Verification items for the finished model (mm, model axes). Round coordinates to 2 decimals unless told otherwise and drop trailing zeros. Write each loop counter-clockwise with the first axis right and the second up, starting at its lowest first coordinate (ties: lowest second). Pieces come first, ordered by that corner, then holes. Notation, with made-up numbers: (13.25, 85.25) -> (25.25, 85.25) arc R29 ccw to (25.25, 116.25) -> close; hole circle Ø1 at (38.25, 26.5). An arc over 180 degrees is marked (long way). Use CSV: the item, a comma, the result in double quotes.
Solid Edge part; units mm, degrees
sketch "Sketch1" plane through (0, 0, 0) normal (0, 0, 1) x (1, 0, 0)
  circle A0 centre (0, 0) radius 4.5
  circle A1 centre (0, 0) radius 2.6
extrude "Protrusion1" add sketch "Sketch1" along normal mid plane 38
fillet "Round_1" radius 0.5 2 edges at (-2.6, 0, -19) (-2.6, 0, 19)
fillet "Round_2" radius 0.5 2 edges at (-4.5, 0, -19) (-4.5, 0, 19)
properties material "Acrylic, high impact grade"
Q1. Mould release check, pull along Y, two halves, no side actions. Record for faces 1 (the flat face through (2, -3, 19)), 2 (the cylindrical face through (-0.338, 2.578, 0.259)), 3 (the cylindrical face through (-0.59, 4.46, 0.26)): released by +Y, released by -Y, zero draft, split by the parting line, or undercut.
Filled in:
face 1,"zero draft"
face 2,"undercut"
face 3,"split by the parting line"
Q2. Section check A-A (x = 0). Record the cut outline in (y, z).
Filled in:
outline,"(-4.5, -18.5) arc R0.5 ccw to (-4, -19) -> (-3.1, -19) arc R0.5 ccw to (-2.6, -18.5) -> (-2.6, 18.5) arc R0.5 ccw to (-3.1, 19) -> (-4, 19) arc R0.5 ccw to (-4.5, 18.5) -> close; (2.6, -18.5) arc R0.5 ccw to (3.1, -19) -> (4, -19) arc R0.5 ccw to (4.5, -18.5) -> (4.5, 18.5) arc R0.5 ccw to (4, 19) -> (3.1, 19) arc R0.5 ccw to (2.6, 18.5) -> close"
Q3. Go/stop test with flat-tipped pins: P1, Ø4, axis at x = 3, z = -6.5, coming from the +Y side; P2, Ø4, axis at y = 3.5, z = -9, coming from the +X side; P3, Ø1.5, axis at x = -2.5, z = -12, coming from the -Y side. Record where each tip stops, or that it passes through.
Filled in:
P1,"y = 4.39"
P2,"x = 4.24"
P3,"y = -4.15"
Q4. Material ranges on L1, parallel to Y at x = 0, z = -10; L2, parallel to Y at x = 0.75, z = 4, recorded low to high.
Filled in:
L1,"-4.5 to -2.6, 2.6 to 4.5"
L2,"-4.44 to -2.49, 2.49 to 4.44"
Q5. Section check C-C (z = -15.5). Record the cut outline in (x, y).
Filled in:
outline,"circle Ø9 at (0, 0); hole circle Ø5.2 at (0, 0)"
